Could you check a few things on this model? Use its own coordinates, in mm. A direction names the side the tool comes from. Round coordinates to 2 decimals unless told otherwise and drop trailing zeros. Loops run counter-clockwise (first coordinate to the right, second up) from the corner with the lowest first, then second, coordinate; pieces in that order, holes last. Notation, with made-up numbers: (47, 62.5) -> (55, 62.5) arc R3 ccw to (55, 67.5) -> close; hole circle Ø4 at (68.25, 86.25). An arc over 180 degrees is marked (long way). Write each question's results on one line, items separated by ' | '.
from build123d import *

# Parameters (mm, degrees)
BOSS_EXTRUDE1_DEPTH = 120
SKETCH2_R           = 40
SKETCH2_R_2         = 3.3
CUT_EXTRUDE1_DEPTH  = 166.743808331
SKETCH3_W           = 15
SKETCH3_H           = 6
CUT_EXTRUDE4_DEPTH  = 86.1
FILLET1_R           = 15
SKETCH4_W           = 24
SKETCH4_H           = 20.775598272
SKETCH4_H_2         = 19.224401728
CUT_EXTRUDE5_DEPTH  = 160.415212574
SKETCH6_W           = 21
SKETCH6_H           = 10
BOSS_EXTRUDE2_DEPTH = 19


with BuildPart() as part:
    # Sketch1 → Boss-Extrude1 (new body)
    with BuildSketch(Plane.XY):
        Polygon((0, 0), (60, 0), (60, 19), (15, 19), (15, 105.1), (0, 105.1), align=None)
    extrude(amount=BOSS_EXTRUDE1_DEPTH)

    # Sketch2 → Cut-Extrude1 (cut, through all)
    with BuildSketch(Plane(origin=(15, 0, 0), x_dir=(0, 0, -1), z_dir=(1, 0, 0))):
        with Locations((-60, 62.05)):
            Circle(SKETCH2_R)
        with Locations((-94.95, 97)):
            Circle(SKETCH2_R_2)
        with Locations((-25.35, 97)):
            Circle(SKETCH2_R_2)
        with Locations(Location((-94.95, 27.1, 0), (0, 0, 180))):
            Circle(SKETCH2_R_2)
        with Locations(Location((-25.35, 27.1, 0), (0, 0, 180))):
            Circle(SKETCH2_R_2)
    extrude(amount=-CUT_EXTRUDE1_DEPTH, mode=Mode.SUBTRACT)

    # Sketch3 → Cut-Extrude4 (cut)
    with BuildSketch(Plane(origin=(0, 19, 0), x_dir=(1, 0, 0), z_dir=(0, 1, 0))):
        with Locations((7.5, -3)):
            Rectangle(SKETCH3_W, SKETCH3_H)
        with Locations((7.5, -117)):
            Rectangle(SKETCH3_W, SKETCH3_H)
    extrude(amount=CUT_EXTRUDE4_DEPTH, mode=Mode.SUBTRACT)

    # Fillet1
    fillet1_edges = [part.edges().sort_by_distance(p)[0] for p in [
        (7.5, 105.1, 6),
        (7.5, 105.1, 114),
    ]]
    fillet(fillet1_edges, radius=FILLET1_R)

    # Sketch4 → Cut-Extrude5 (cut, through all)
    with BuildSketch(Plane(origin=(0, 19, 0), x_dir=(1, 0, 0), z_dir=(0, 1, 0))):
        with Locations((48, -109.612200864)):
            Rectangle(SKETCH4_W, SKETCH4_H)
        with Locations((48, -9.612200864)):
            Rectangle(SKETCH4_W, SKETCH4_H_2)
    extrude(amount=-CUT_EXTRUDE5_DEPTH, mode=Mode.SUBTRACT)

    # Sketch6 → Boss-Extrude2 (add)
    with BuildSketch(Plane(origin=(0, 19, 0), x_dir=(1, 0, 0), z_dir=(0, 1, 0))):
        with Locations((25.5, 5)):
            Rectangle(SKETCH6_W, SKETCH6_H)
        with Locations((25.5, -125)):
            Rectangle(SKETCH6_W, SKETCH6_H)
    extrude(amount=-BOSS_EXTRUDE2_DEPTH)


solid = part.part
1) If we mould it in two halves opening along Y, with no side actions, what happens to faces 1 (the cylindrical face through (7.6, 99.23, 97.38)), 2 (the flat face through (30, 19, 59)), 3 (the flat face through (48, 10, 99.224)), 4 (the flat face through (30, 0, 59))? For each: released by +Y, released by -Y, zero draft, split by the parting line, or undercut.
Model answer:
face 1: undercut | face 2: released by +Y | face 3: zero draft | face 4: released by -Y
2) For faces 5 (the flat face through (15, 23, 47)), 6 (the flat face through (7, 10, 0)), 7 (the flat face through (36, 10, 5)), 8 (the flat face through (7, 54, 6)), 9 (the flat face through (7, 10, 120)), which set-ups out of +Z, -Z, +X, -X, +Y, -Y let a thin tool reach every point of the face, with its end or its side?
Model answer:
face 5: +Z, -Z, +X, +Y | face 6: -Z, -X, +Y, -Y | face 7: -Z, +X, +Y, -Y | face 8: -Z, +X, -X, +Y | face 9: +Z, -X, +Y, -Y
3) I want a section at A-A, the plane x = 9. Write out the boundary of the cut face in (y, z), plus the area to 3 significant figures.
Model answer:
outline: (0, 0) -> (19, 0) -> (19, 6) -> (90.1, 6) arc R15 ccw to (105.1, 21) -> (105.1, 99) arc R15 ccw to (90.1, 114) -> (19, 114) -> (19, 120) -> (0, 120) -> close; hole circle Ø80 at (62.05, 60); hole circle Ø6.6 at (27.1, 25.35); hole circle Ø6.6 at (27.1, 94.95); hole circle Ø6.6 at (97, 25.35); hole circle Ø6.6 at (97, 94.95) | area: 6,320 mm2
4) I want a section at D-D, the plane y = 62.05. Write out the boundary of the cut face in (x, z).
Model answer:
outline: (0, 6) -> (15, 6) -> (15, 20) -> (0, 20) -> close; (0, 100) -> (15, 100) -> (15, 114) -> (0, 114) -> close
5) I need wall thicknesses on line 1 (Z direction, x = 6, y = 27); line 2 (Y direction, x = 4.5, z = 60); line 3 (Y direction, x = 5.25, z = 25.35). Which ranges of each line are inside material? Lowest first, please.
Model answer:
line 1: z = 6 to 22.05, 28.65 to 40.73, 79.27 to 91.65, 98.25 to 114 | line 2: y = 0 to 22.05, 102.05 to 105.1 | line 3: y = 0 to 23.8, 30.4 to 42.07, 82.03 to 93.7, 100.3 to 105.1
6) I want a section at C-C, the plane y = 97. Write out the boundary of the cut face in (x, z), plus the area to 3 significant figures.
Model answer:
outline: (0, 7.68) -> (15, 7.68) -> (15, 22.05) -> (0, 22.05) -> close; (0, 28.65) -> (15, 28.65) -> (15, 40.54) -> (0, 40.54) -> close; (0, 79.46) -> (15, 79.46) -> (15, 91.65) -> (0, 91.65) -> close; (0, 98.25) -> (15, 98.25) -> (15, 112.32) -> (0, 112.32) -> close | area: 788 mm2
7) I'm going to push flat-ended pins straight in: pin 1 (8.5 mm diameter, centred on y = 27.1, z = 25.35, fed in from +X); pin 2 (15 mm diameter, centred on y = 8.5, z = 116, fed in from +X); pin 3 (2 mm diameter, centred on x = 8, y = 21, fed in from +Z). Where does each tip first touch, or does it pass through?
Model answer:
pin 1: stops at x = 15 | pin 2: stops at x = 36 | pin 3: stops at z = 114
8) I want a section at B-B, the plane z = 60. Write out the boundary of the cut face in (x, y), plus the area to 3 significant figures.
Model answer:
outline: (0, 0) -> (60, 0) -> (60, 19) -> (15, 19) -> (15, 22.05) -> (0, 22.05) -> close; (0, 102.05) -> (15, 102.05) -> (15, 105.1) -> (0, 105.1) -> close | area: 1,230 mm2
